Verification items for the finished model (mm, model axes). Face numbers are marked on the shaded views. Coordinates: 2 decimals unless noted, no trailing zeros. Write each loop counter-clockwise with the first axis right and the second up, starting at its lowest first coordinate (ties: lowest second). Pieces come first, ordered by that corner, then holes. Notation, with made-up numbers: (10.5, -32.5) - (17.5, -32.5) arc R35 cw to (17.5, 2.5) - close; hole circle Ø9 at (68, 6.5). An arc over 180 degrees is marked (long way). Use CSV: the item, a comma, the result in double quotes. Start each with the question number.
```python
from build123d import *

# Parameters (mm, degrees)
SKETCH1_W          = 88.9
SKETCH1_H          = 12.7
BASE_FLANGE1_DEPTH = 0.7
EDGE_FLANGE1_DEPTH = 88.9
EDGE_FLANGE2_DEPTH = 88.9


# Sheet-metal steps are written as plain solids
with BuildPart() as part:
    # Sketch1 → Base-Flange1 (new body)
    with BuildSketch(Plane(origin=(0, 0, 0), x_dir=(1, 0, 0), z_dir=(0, 1, 0))):
        Rectangle(SKETCH1_W, SKETCH1_H)
    extrude(amount=-BASE_FLANGE1_DEPTH)

    # Edge-Flange1 section (across the edge) → Edge-Flange1 (add)
    with BuildSketch(Plane(origin=(44.45, 0, -8.15), x_dir=(0, 0, 1), z_dir=(-1, 0, 0))):
        with BuildLine():
            Line((-0.7, 1), (-0.7, 152.4))
            Line((-0.7, 152.4), (0, 152.4))
            Line((0, 152.4), (0, 1))
            ThreePointArc((0, 1), (0.292893219, 0.292893219), (1, 0))
            Line((1, 0), (1.8, 0))
            Line((1.8, 0), (1.8, -0.7))
            Line((1.8, -0.7), (1, -0.7))
            ThreePointArc((1, -0.7), (-0.202081528, -0.202081528), (-0.7, 1))
        make_face()
    extrude(amount=EDGE_FLANGE1_DEPTH)

    # Edge-Flange2 section (across the edge) → Edge-Flange2 (add)
    with BuildSketch(Plane(origin=(44.45, 152.814213562, -8.15), x_dir=(0, -0.7071067811865414, 0.7071067811865537), z_dir=(-1, 0, 0))):
        with BuildLine():
            Line((-0.7, 0.414213562), (-0.7, 35.9156))
            Line((-0.7, 35.9156), (0, 35.9156))
            Line((0, 35.9156), (0, 0.414213562))
            ThreePointArc((0, 0.414213562), (0.076120467, 0.03153013), (0.292893219, -0.292893219))
            Line((0.292893219, -0.292893219), (-0.202081528, -0.787867966))
            ThreePointArc((-0.202081528, -0.787867966), (-0.570595205, -0.236348273), (-0.7, 0.414213562))
        make_face()
    extrude(amount=EDGE_FLANGE2_DEPTH)


solid = part.part
```
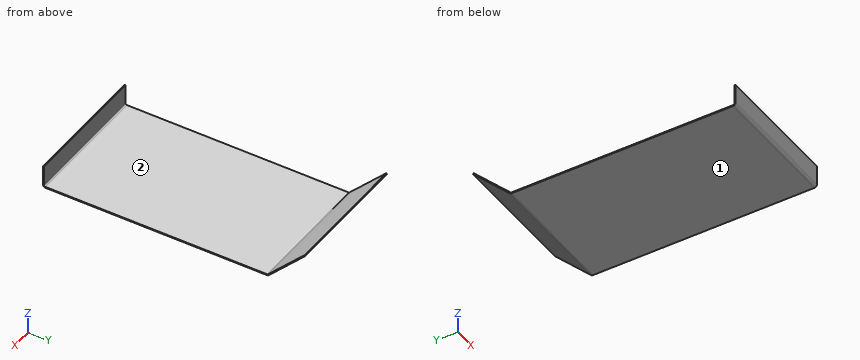
Q1. Cross-section at A-A (x = 33.5). Record the cut outline in (y, z).
Q2. Release check for a two-part mould opening along Y. For the marked faces 1 and 2 record: released by +Y, released by -Y, zero draft, split by the parting line, or undercut.
Q3. Cross-section at B-B (z = -3.75). Record the cut outline in (x, y).
Q4. Cross-section at C-C (y = 113). Record the cut outline in (x, z), plus the area to 3 significant figures.
Q5. Scan lines: line 1 along Z through (x, y) = (-27, 45); line 2 along Y through (x, z) = (14, 3); line 3 along Y through (x, z) = (-26.5, 3.5). Record each from-to range of solid material in increasing order. Write a range as from..to.
Q6. Cross-section at D-D (z = 12). Record the cut outline in (x, y), plus the area to 3 significant figures.
Q7. Gauge pin test, flat ends, axial feed: pin 1 (0.6 mm diameter, centred on x = -2, y = 0, fed in from +Z); pin 2 (8 mm diameter, centred on x = 22, y = 31, fed in from +Z); pin 3 (12 mm diameter, centred on x = -28.5, z = 10, fed in from +Y). Record the tip position at first contact, or that the pin passes through.
Reply:
1,outline,"(-0.7, -7.15) arc R1.7 ccw to (1, -8.85) - (152.4, -8.85) arc R1.7 ccw to (153.6, -8.35) - (178.71, 16.75) - (178.21, 17.25) - (153.11, -7.86) arc R1 cw to (152.4, -8.15) - (1, -8.15) arc R1 cw to (0, -7.15) - (0, 6.35) - (-0.7, 6.35) - close"
2,face 1,"zero draft"
2,face 2,"undercut"
3,outline,"(-44.45, -0.7) - (44.45, -0.7) - (44.45, 0) - (-44.45, 0) - close; (-44.45, 157.21) - (44.45, 157.21) - (44.45, 158.2) - (-44.45, 158.2) - close"
4,outline,"(-44.45, -8.85) - (44.45, -8.85) - (44.45, -8.15) - (-44.45, -8.15) - close"
4,area,"62.2 mm^2"
5,line 1,"-8.85..-8.15"
5,line 2,"-0.7..0, 163.96..164.95"
5,line 3,"-0.7..0, 164.46..165.45"
6,outline,"(-44.45, 172.96) - (44.45, 172.96) - (44.45, 173.95) - (-44.45, 173.95) - close"
6,area,"88.0 mm^2"
7,pin 1,"z = 6.35"
7,pin 2,"z = -8.15"
7,pin 3,"y = 177.95"
